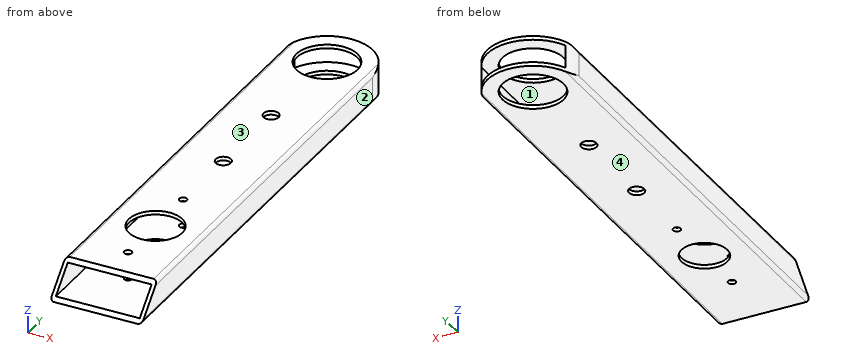
```python
from build123d import *

# Parameters (mm, degrees)
SKETCH1_W           = 34.925
SKETCH1_H           = 9.525
BOSS_EXTRUDE1_DEPTH = 203.2
SKETCH2_R           = 3.175
SKETCH2_R_2         = 12.7
SKETCH2_R_3         = 1.5875
SKETCH2_R_4         = 9.525
CUT_EXTRUDE1_DEPTH  = 13.7
CUT_EXTRUDE2_DEPTH  = 39.1000001
SKETCH4_R           = 11.1125
CUT_EXTRUDE3_DEPTH  = 1.5875


with BuildPart() as part:
    # Sketch1 → Boss-Extrude1 (new body)
    with BuildSketch(Plane(origin=(0, 0, 0), x_dir=(1, 0, 0), z_dir=(0, 1, 0))):
        with BuildLine():
            Line((1.5875, 0), (36.5125, 0))
            ThreePointArc((36.5125, 0), (37.635032015, 0.464967985), (38.1, 1.5875))
            Line((38.1, 1.5875), (38.1, 11.1125))
            ThreePointArc((38.1, 11.1125), (37.635032015, 12.235032015), (36.5125, 12.7))
            Line((36.5125, 12.7), (1.5875, 12.7))
            ThreePointArc((1.5875, 12.7), (0.464967985, 12.235032015), (0, 11.1125))
            Line((0, 11.1125), (0, 1.5875))
            ThreePointArc((0, 1.5875), (0.464967985, 0.464967985), (1.5875, 0))
        make_face()
        with Locations((19.05, 6.35)):
            Rectangle(SKETCH1_W, SKETCH1_H, mode=Mode.SUBTRACT)
    extrude(amount=BOSS_EXTRUDE1_DEPTH)

    # Sketch2 → Cut-Extrude1 (cut, through all)
    with BuildSketch(Plane.XY):
        with Locations((19.05, 101.6)):
            Circle(SKETCH2_R)
        with Locations((19.05, 139.7)):
            Circle(SKETCH2_R)
        with Locations((19.05, 184.15)):
            Circle(SKETCH2_R_2)
        with Locations((19.05, 25.704689783)):
            Circle(SKETCH2_R_3)
        with Locations((19.05, 47.625)):
            Circle(SKETCH2_R_4)
        with Locations((19.05, 69.545310217)):
            Circle(SKETCH2_R_3)
        with BuildLine():
            Line((0, 184.15), (0, 209.55))
            Line((0, 209.55), (38.1, 209.55))
            Line((38.1, 209.55), (38.1, 184.15))
            ThreePointArc((38.1, 184.15), (19.05, 203.2), (0, 184.15))
        make_face()
    extrude(amount=-CUT_EXTRUDE1_DEPTH, mode=Mode.SUBTRACT)

    # Sketch3 → Cut-Extrude2 (cut, through all)
    with BuildSketch(Plane(origin=(38.1, 0, 0), x_dir=(0, 0, -1), z_dir=(1, 0, 0))):
        Polygon((0, 0), (12.7, 0), (0, 12.7), align=None)
    extrude(amount=-CUT_EXTRUDE2_DEPTH, mode=Mode.SUBTRACT)

    # Sketch4 → Cut-Extrude3 (cut)
    with BuildSketch(Plane.XY):
        with Locations((19.05, 47.625)):
            Circle(SKETCH4_R)
    extrude(amount=-CUT_EXTRUDE3_DEPTH, mode=Mode.SUBTRACT)


solid = part.part
```
Verification items for the finished model (mm, model axes). Face numbers are marked on the shaded views. Coordinates: 2 decimals unless noted, no trailing zeros. Loops run counter-clockwise (first coordinate to the right, second up) from the corner with the lowest first, then second, coordinate; pieces in that order, holes last. Notation, with made-up numbers: (73, 70.5) - (112, 70.5) arc R28 ccw to (112, 96.5) - close; hole circle Ø6 at (-15, 50). An arc over 180 degrees is marked (long way). Return JSON: item names as keys, results as strings.
1. Section check D-D, the plane x = 34.5. Record the boundary of the cut face in (y, z), then the cut area to 3 significant figures.
Established:
{"outline": "(0, -12.7) - (195.29, -12.7) - (195.29, -11.11) - (1.59, -11.11) - close; (11.11, -1.59) - (195.29, -1.59) - (195.29, 0) - (12.7, 0) - close", "area": "600 mm2"}
2. Section check A-A, the plane y = 139.7. Record the boundary of the cut face in (x, z) (1 decimal), then the cut area to 3 significant figures.
Established:
{"outline": "(0, -11.1) arc R1.6 ccw to (1.6, -12.7) - (15.9, -12.7) - (15.9, -11.1) - (1.6, -11.1) - (1.6, -1.6) - (15.9, -1.6) - (15.9, 0) - (1.6, 0) arc R1.6 ccw to (0, -1.6) - close; (22.2, -12.7) - (36.5, -12.7) arc R1.6 ccw to (38.1, -11.1) - (38.1, -1.6) arc R1.6 ccw to (36.5, 0) - (22.2, 0) - (22.2, -1.6) - (36.5, -1.6) - (36.5, -11.1) - (22.2, -11.1) - close", "area": "129 mm2"}
3. Thickness scan on L1, parallel to X at y = 154, z = -2.25; L2, parallel to Z at x = 5, y = 60.5; L3, parallel to X at y = 164, z = -1.5. Record the ranges inside material, lowest first.
Established:
{"L1": "x = 0 to 1.59, 36.51 to 38.1", "L2": "z = -12.7 to -11.11, -1.59 to 0", "L3": "x = 0 to 38.1"}
4. Section check C-C, the plane y = 87.5. Record the boundary of the cut face in (x, z) (1 decimal), then the cut area to 3 significant figures.
Established:
{"outline": "(0, -11.1) arc R1.6 ccw to (1.6, -12.7) - (36.5, -12.7) arc R1.6 ccw to (38.1, -11.1) - (38.1, -1.6) arc R1.6 ccw to (36.5, 0) - (1.6, 0) arc R1.6 ccw to (0, -1.6) - close; hole (1.6, -11.1) - (36.5, -11.1) - (36.5, -1.6) - (1.6, -1.6) - close", "area": "149 mm2"}
5. Section check B-B, the plane z = -8.5. Record the boundary of the cut face in (x, y).
Established:
{"outline": "(0, 4.2) - (1.59, 4.2) - (1.59, 191.76) arc R19.05 ccw to (0, 184.15) - close; (36.51, 4.2) - (38.1, 4.2) - (38.1, 184.15) arc R19.05 ccw to (36.51, 191.76) - close"}
6. Go/stop test with flat-tipped pins: pin 1 (4 mm diameter, centred on x = 14.5, z = -3, fed in from +Y); pin 2 (1.9 mm diameter, centred on x = 19.05, y = 69.55, fed in from -Z). Record where each tip stops, or that it passes through.
Established:
{"pin 1": "stops at y = 202.94", "pin 2": "passes through"}
7. Mould release check, pull along Z, two halves, no side actions. Record for the marked faces 1, 2, 3 and 4: +Z half, -Z half, draft (parallel to the pull), parting line (faces both ways), or undercut.
Established:
{"face 1": "undercut", "face 2": "draft", "face 3": "+Z half", "face 4": "-Z half"}
